Geometry check sheet. Reference: drawing and pictorial views, mm from the part's lowest x, y, z. A direction names the side the tool comes from. Coordinates: 2 decimals unless noted, no trailing zeros. Write each loop counter-clockwise with the first axis right and the second up, starting at its lowest first coordinate (ties: lowest second). Pieces come first, ordered by that corner, then holes. Notation, with made-up numbers: (60, 21) - (108, 21) arc R21 ccw to (108, 31) - close; hole circle Ø2 at (26.25, 80). An arc over 180 degrees is marked (long way). Answer as CSV lines item,"result". Start each with the question number.
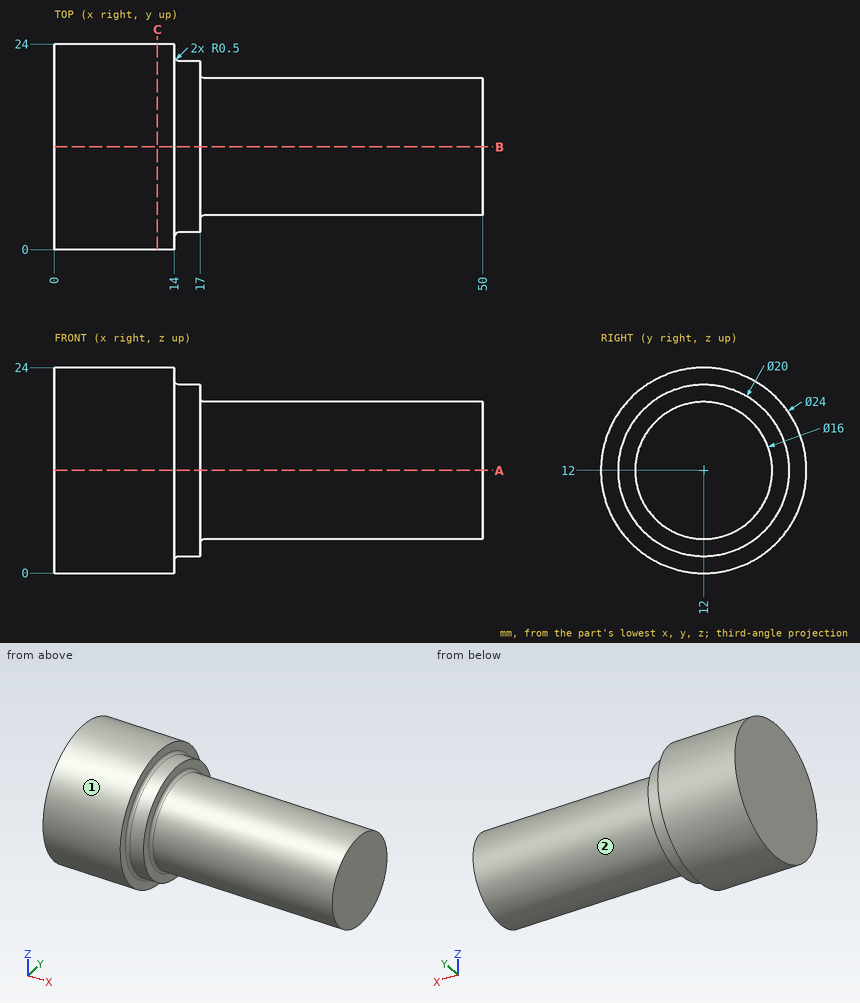
1. Cross-section at C-C (x = 12). Record the cut outline in (y, z), and give its area (3 significant figures).
2. Access from +Z, -Z, +X, -X, +Y, -Y to the whole of each face (thin tool, end or side, straight path). Record for the marked faces 1 and 2.
3. Depth check by flat-ended pin: P1, Ø3, axis at x = 38.5, z = 15.5, coming from the -Y side; P2, Ø1.5, axis at x = 23.5, z = 9.5, coming from the -Y side; P3, Ø8, axis at x = 44, y = 20.5, coming from the +Z side. Enter the tip coordinate at first touch or a pass-through.
4. Scan lines: line 1 along X through (y, z) = (2, 8.5); line 2 along X through (y, z) = (12.5, 21.75); line 3 along Z through (x, y) = (24, 17.5). Record each from-to range of solid material in increasing order. Write a range as from..to.
5. Cross-section at A-A (z = 12). Record the cut outline in (x, y).
Completed:
1,outline,"circle Ø24 at (12, 12)"
1,area,"452 mm2"
2,face 1,"+X, -X"
2,face 2,"+X"
3,P1,"stops at y = 4.25"
3,P2,"stops at y = 4.19"
3,P3,"stops at z = 18.61"
4,line 1,"x = 0..14"
4,line 2,"x = 0..17"
4,line 3,"z = 6.19..17.81"
5,outline,"(0, 0) - (14, 0) - (14, 1.5) arc R0.5 cw to (14.5, 2) - (17, 2) - (17, 3.5) arc R0.5 cw to (17.5, 4) - (50, 4) - (50, 20) - (17.5, 20) arc R0.5 cw to (17, 20.5) - (17, 22) - (14.5, 22) arc R0.5 cw to (14, 22.5) - (14, 24) - (0, 24) - close"
